from build123d import *

# Parameters (mm, degrees)
EXTRUDE_1_DEPTH     = 3
SKETCH_2_R          = 1.575
SKETCH_2_R_2        = 6.8
CUT_EXTRUDE_2_DEPTH = 59.386642308
FILLET_1_R          = 5


with BuildPart() as part:
    # 草图1 → 凸台-拉伸1 (new body)
    with BuildSketch(Plane.XY):
        Polygon((0, 0), (0, -20), (5, -50), (25, -50), (30, -20), (30, 0), align=None)
    extrude(amount=EXTRUDE_1_DEPTH)

    # 草图2 → 切除-拉伸2 (cut, through all)
    with BuildSketch(Plane.XY.offset(3)):
        with Locations(Location((10, -5, 0), (0, 0, 180))):
            Circle(SKETCH_2_R)
        with Locations((10, -15)):
            Circle(SKETCH_2_R)
        with Locations(Location((20, -15, 0), (0, 0, 180))):
            Circle(SKETCH_2_R)
        with Locations((20, -5)):
            Circle(SKETCH_2_R)
        with Locations((15, -35)):
            Circle(SKETCH_2_R_2)
        with Locations((15, -25.5)):
            Circle(SKETCH_2_R)
        with Locations((23.227241336, -39.75)):
            Circle(SKETCH_2_R)
        with Locations((6.772758664, -39.75)):
            Circle(SKETCH_2_R)
    extrude(amount=-CUT_EXTRUDE_2_DEPTH, mode=Mode.SUBTRACT)

    # 圆角1
    fillet_1_edges = [part.edges().sort_by_distance(p)[0] for p in [
        (30, 0, 1.5),
        (30, -20, 1.5),
        (25, -50, 1.5),
        (5, -50, 1.5),
        (0, -20, 1.5),
        (0, 0, 1.5),
    ]]
    fillet(fillet_1_edges, radius=FILLET_1_R)


solid = part.part
The listing builds one solid part. Answer for the finished solid, in the listing's coordinates (mm). Round coordinates to 2 decimals unless told otherwise and drop trailing zeros. Loops run counter-clockwise (first coordinate to the right, second up) from the corner with the lowest first, then second, coordinate; pieces in that order, holes last. Notation, with made-up numbers: M 33.5,42 L 87.5,42 A33 cw 87.5,77 Z; hole C 40,13.25 d9. An arc over 180 degrees is marked long. Return JSON: item names as keys, results as strings.
Q1. Find the intervals of material crossed by line 1 along Y through (x, z) = (15, 1.85) (3 decimals); line 2 along Y through (x, z) = (10, 1.55) (3 decimals); line 3 along Y through (x, z) = (9, 0.2), in increasing order. Write a range as from..to.
Results list:
{"line 1": "y = -50..-41.8, -28.2..-27.075, -23.925..0", "line 2": "y = -50..-39.609, -30.391..-16.575, -13.425..-6.575, -3.425..0", "line 3": "y = -49.99..-38.2, -31.8..-16.22, -13.78..-6.22, -3.78..0"}
Q2. Find section C-C, the plane y = -35. Determine the outline of the cut face in (x, z), plus the area to 3 significant figures.
Results list:
{"outline": "M 2.5,0 L 8.2,0 L 8.2,3 L 2.5,3 Z; M 21.8,0 L 27.5,0 L 27.5,3 L 21.8,3 Z", "area": "34.2 mm2"}
Q3. Find section D-D, the plane x = 10. Determine the outline of the cut face in (y, z) (3 decimals), plus the area to 3 significant figures.
Results list:
{"outline": "M -50,0 L -39.609,0 L -39.609,3 L -50,3 Z; M -30.391,0 L -16.575,0 L -16.575,3 L -30.391,3 Z; M -13.425,0 L -6.575,0 L -6.575,3 L -13.425,3 Z; M -3.425,0 L 0,0 L 0,3 L -3.425,3 Z", "area": "103 mm2"}
Q4. Each of these flat-tipped pins is pushed along its axis until it touches: pin 1 Ø1 at (y, z) = (-40.5, 0.5) entering from +X; pin 2 Ø4 at (x, y) = (20, -5) entering from -Z. Where does it stop, or does it pass through?
Results list:
{"pin 1": "stops at x = 26.67", "pin 2": "stops at z = 0"}
Q5. Find section B-B, the plane y = -15. Determine the outline of the cut face in (x, z) (3 decimals).
Results list:
{"outline": "M 0,0 L 8.425,0 L 8.425,3 L 0,3 Z; M 11.575,0 L 18.425,0 L 18.425,3 L 11.575,3 Z; M 21.575,0 L 30,0 L 30,3 L 21.575,3 Z"}
Q6. The mould has two halves that part along Y. Classify faces 1 (the face through (21.281, -37.604, 1.521)), 2 (the face through (30, -12, 1)), 3 (the face through (15, 0, 1)): released by +Y, released by -Y, zero draft, split by the parting line, or undercut.
Results list:
{"face 1": "undercut", "face 2": "zero draft", "face 3": "released by +Y"}
Q7. Find section A-A, the plane z = 1.05. State how many separate pieces and enclosed holes the cut face has, plus the area to 3 significant figures.
Results list:
{"separate pieces": "1", "enclosed holes": "8", "area": "1,130 mm2"}
